from build123d import *

# Parameters (mm, degrees)
EXTRUDE_1_DEPTH             = 10
HOLE_WIZARD_M4_1_D          = 3.3
HOLE_WIZARD_M4_1_DEPTH      = 7.999993258
CUT_EXTRUDE_1_DEPTH         = 5
SKETCH_6_W                  = 85
SKETCH_6_H                  = 65
EXTRUDE_2_DEPTH             = 5
SKETCH_7_W                  = 15
SKETCH_7_H                  = 15
CUT_EXTRUDE_2_DEPTH         = 5
PATTERN_LINEAR_1_COUNT      = 4
PATTERN_LINEAR_1_PITCH      = 20
PATTERN_LINEAR_1_COUNT_DIR2 = 3
PATTERN_LINEAR_1_PITCH_DIR2 = 20


with BuildPart() as part:
    # 草图1 → 凸台-拉伸1 (new body)
    with BuildSketch(Plane.XY):
        Polygon((0.020144186, -0.052366179), (0.016918395, 5.947632954), (-29.983056322, 5.986581065), (-29.962376808, 12.486559695), (0.03759791, 12.447611584), (0.03759791, 20.447611584), (-29.962376808, 20.486559695), (-40.315163894, 20.486559695), (-40.315163894, 0), align=None)
    extrude(amount=EXTRUDE_1_DEPTH)

    # M4 螺纹孔的螺纹孔钻头1
    with Locations(Plane(origin=(0.026546569, 20.447625932, 0), x_dir=(0.999999157, -0.00129827, 0), z_dir=(0.00129827, 0.999999157, 0))):
        with Locations((-15, -5), (-5, -5)):
            Hole(HOLE_WIZARD_M4_1_D / 2, depth=HOLE_WIZARD_M4_1_DEPTH)

    # 草图5 → 切除-拉伸1 (cut)
    with BuildSketch(Plane(origin=(0.016160415, 12.447639416, 0), x_dir=(0.999999157, -0.00129827, 0), z_dir=(-0.00129827, -0.999999157, 0))):
        with BuildLine():
            Line((-16.077032961, 2.2), (-13.922967039, 2.2))
            ThreePointArc((-13.922967039, 2.2), (-12, 5), (-13.922967039, 7.8))
            Line((-13.922967039, 7.8), (-16.077032961, 7.8))
            ThreePointArc((-16.077032961, 7.8), (-18, 5), (-16.077032961, 2.2))
        make_face()
        with BuildLine():
            Line((-6.077032961, 2.2), (-3.922967039, 2.2))
            ThreePointArc((-3.922967039, 2.2), (-2, 5), (-3.922967039, 7.8))
            Line((-3.922967039, 7.8), (-6.077032961, 7.8))
            ThreePointArc((-6.077032961, 7.8), (-8, 5), (-6.077032961, 2.2))
        make_face()
    extrude(amount=-CUT_EXTRUDE_1_DEPTH, mode=Mode.SUBTRACT)

    # 草图6 → 凸台-拉伸2 (add)
    with BuildSketch(Plane.XY):
        with Locations((-82.815163894, 19.23657038)):
            Rectangle(SKETCH_6_W, SKETCH_6_H)
    extrude(amount=EXTRUDE_2_DEPTH)

    # 草图7 → 切除-拉伸2 (cut)
    with BuildSketch(Plane.XY.offset(5)):
        with Locations((-112.815163894, 39.23657038)):
            Rectangle(SKETCH_7_W, SKETCH_7_H)
    cut_extrude_2 = extrude(amount=-CUT_EXTRUDE_2_DEPTH, mode=Mode.SUBTRACT)

    # 阵列(线性)1: Cut-Extrude 2 4 × 3
    with Locations(*[(i * PATTERN_LINEAR_1_PITCH, -j * PATTERN_LINEAR_1_PITCH_DIR2, 0) for i in range(PATTERN_LINEAR_1_COUNT) for j in range(PATTERN_LINEAR_1_COUNT_DIR2) if (i, j) != (0, 0)]):
        add(cut_extrude_2, mode=Mode.SUBTRACT)


solid = part.part
The model under review builds one solid part; all positions refer to its coordinate system, in mm. A direction names the side the tool comes from. Give positions to 0.01 mm unless a question says otherwise; leave off trailing zeros. Order: outer loops, then holes, each group sorted by start corner. A loop starts at its lowest first (then second) coordinate and runs counter-clockwise, first axis right, second up. Notation, with made-up numbers: (80.25, -22) -> (109.25, -22) arc R20 cw to (109.25, -5) -> close; hole circle Ø6 at (-22.75, 72.25). An arc over 180 degrees is marked (long way). Write item = value, one per line. Start each with the question number.
(1) Take a section at D-D (y = 2). Write out the cut boundary in (x, z).
(2) Take a section at B-B (x = -96). Write out the cut boundary in (y, z), plus the area to 3 significant figures.
(3) Draft analysis for pull direction Y (two halves, no side actions). For faces 1 (the flat face through (-20, 13, 10)), 2 (the flat face through (-83, -13.263, 2)), 3 (the flat face through (-53, 11.737, 3)), state which applies: +Y half, -Y half, draft (parallel to the pull), parting line (faces both ways), or undercut.
(4) Take a section at C-C (x = -24.5). Write out the cut boundary in (y, z), plus the area to 3 significant figures.
(5) For pin 1 Ø10 at (x, y) = (-60.5, 25) entering from +Z; pin 2 Ø3 at (x, y) = (-58.5, 37) entering from +Z; pin 3 Ø4 at (y, z) = (37.5, 2) entering from +X; pin 4 Ø5 at (x, z) = (-17, 6) entering from -Y, all flat-tipped, find the tip position at first contact; note any pin that passes through.
(6) Take a section at A-A (y = 36.5). Write out the cut boundary in (x, z), plus the area to 3 significant figures.
(7) Tool access review of faces 4 (the flat face through (-40.315, 10, 7)), 5 (the flat face through (-73, 6.737, 3)): name each direction out of +Z, -Z, +X, -X, +Y, -Y from which nothing blocks a thin tool from reaching the whole face with its end or side.
(8) For L1, parallel to X at y = 1, z = 1.25; L2, parallel to X at y = 46, z = 0.75; L3, parallel to Y at x = -58.5, z = 1.25, list the stretches that pass through material, from the lowest coordinate up. Write a range as from..to.
Returned:
q1.outline = (-125.32, 0) -> (-120.32, 0) -> (-120.32, 5) -> (-125.32, 5) -> close; (-105.32, 0) -> (-100.32, 0) -> (-100.32, 5) -> (-105.32, 5) -> close; (-85.32, 0) -> (-80.32, 0) -> (-80.32, 5) -> (-85.32, 5) -> close; (-65.32, 0) -> (-60.32, 0) -> (-60.32, 5) -> (-65.32, 5) -> close; (-45.32, 0) -> (0.02, 0) -> (0.02, 10) -> (-40.32, 10) -> (-40.32, 5) -> (-45.32, 5) -> close
q2.outline = (-13.26, 0) -> (-8.26, 0) -> (-8.26, 5) -> (-13.26, 5) -> close; (6.74, 0) -> (11.74, 0) -> (11.74, 5) -> (6.74, 5) -> close; (26.74, 0) -> (31.74, 0) -> (31.74, 5) -> (26.74, 5) -> close; (46.74, 0) -> (51.74, 0) -> (51.74, 5) -> (46.74, 5) -> close
q2.area = 100 mm²
q3.face_1 = draft
q3.face_2 = -Y half
q3.face_3 = undercut
q4.outline = (-0.02, 0) -> (5.98, 0) -> (5.98, 10) -> (-0.02, 10) -> close; (12.48, 0) -> (20.48, 0) -> (20.48, 10) -> (12.48, 10) -> close
q4.area = 140 mm²
q5.pin_1 = 5
q5.pin_2 = through
q5.pin_3 = -40.32
q5.pin_4 = -0.03
q6.outline = (-125.32, 0) -> (-120.32, 0) -> (-120.32, 5) -> (-125.32, 5) -> close; (-105.32, 0) -> (-100.32, 0) -> (-100.32, 5) -> (-105.32, 5) -> close; (-85.32, 0) -> (-80.32, 0) -> (-80.32, 5) -> (-85.32, 5) -> close; (-65.32, 0) -> (-60.32, 0) -> (-60.32, 5) -> (-65.32, 5) -> close; (-45.32, 0) -> (-40.32, 0) -> (-40.32, 5) -> (-45.32, 5) -> close
q6.area = 125 mm²
q7.face_4 = +Z, -X, +Y, -Y
q7.face_5 = +Z, -Z
q8.L1 = -125.32..-120.32, -105.32..-100.32, -85.32..-80.32, -65.32..-60.32, -45.32..0.02
q8.L2 = -125.32..-120.32, -105.32..-100.32, -85.32..-80.32, -65.32..-60.32, -45.32..-40.32
q8.L3 = -13.26..-8.26, 6.74..11.74, 26.74..31.74, 46.74..51.74
